Geometry: see drawing. Coordinates: mm, zero at the bounding-box minimum. A direction names the side the tool comes from. Give positions to 0.01 mm unless a question says otherwise; leave off trailing zeros. Order: outer loops, then holes, each group sorted by start corner. A loop starts at its lowest first (then second) coordinate and runs counter-clockwise, first axis right, second up. Notation, with made-up numbers: (-2, 8) - (28, 8) arc R20 cw to (28, 29) - close; hole circle Ø5 at (85.5, 56). An arc over 180 degrees is marked (long way). Put each result on its own line as item: value. Start each with the question number.
1. Set-up query: the marked faces 4, 5 and 6. Return all of +Z, -Z, +X, -X, +Y, -Y with unobstructed straight access to the full face (end or side cutting, diameter ignored); none if empty.
2. Section D-D on y = 4.6. Return the cut outline in (x, z) (1 decimal).
3. Mould query, pull axis Y, two halves, no side actions, for the marked faces 1, 2 and 3. Classes: pulls with the +Y half, pulls with the -Y half, needs draft (parallel to the pull), parting line crosses it, or undercut.
4. Section C-C on z = 7.25. Return the cut outline in (x, y).
5. Ray query, line 1 along Z through (x, y) = (4.5, 1.9); line 2 along Y through (x, z) = (3.55, 11.5); line 3 along Y through (x, z) = (2.4, 12). Return the intervals inside material, ascending. Write a range as from..to.
6. Section B-B on x = 3.1. Return the cut outline in (y, z).
7. First-contact query: P1, Ø2, axis at y = 4, z = 8, coming from the -X side; P2, Ø1.5, axis at y = 1, z = 11.5, coming from the +X side. Flat tips, straight axial feed; report the tip coordinate or a pass-through.
8. Section A-A on y = 2.75. Return the cut outline in (x, z).
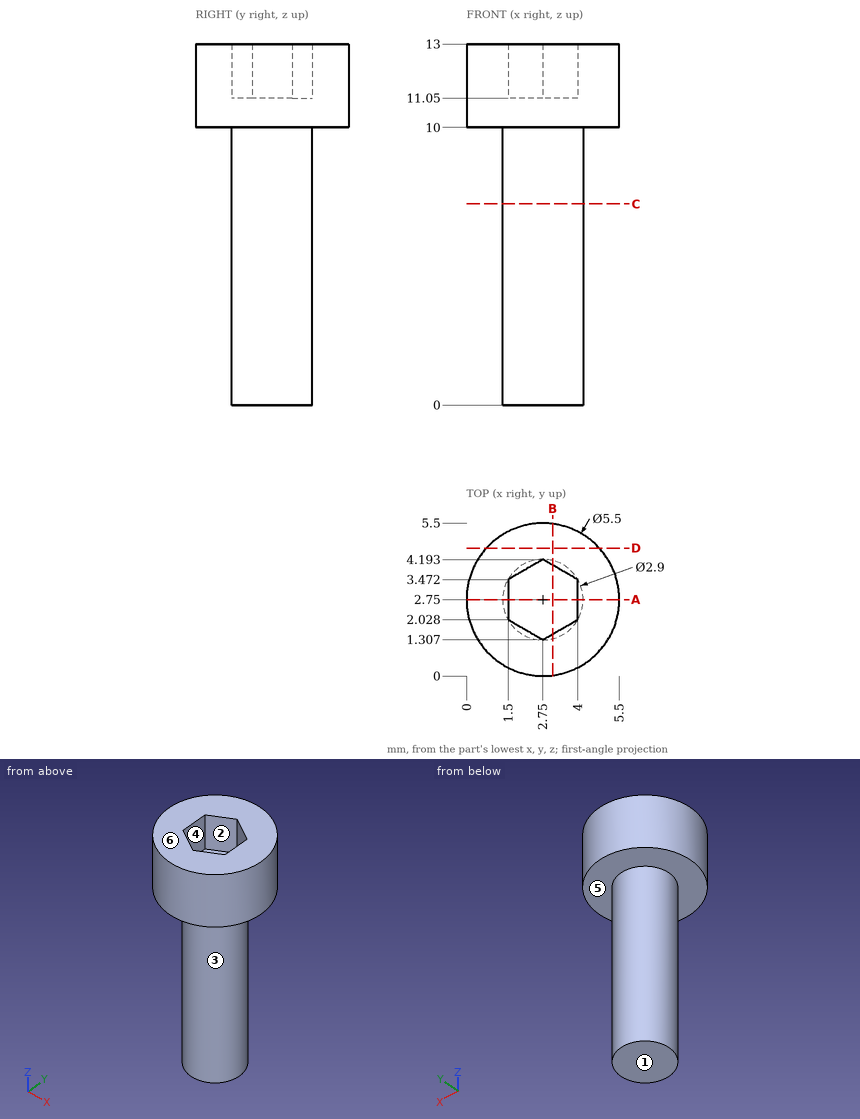
Resolved:
1. face 4: +Z
1. face 5: -Z
1. face 6: +Z, +X, -X, +Y, -Y
2. outline: (0.7, 10) - (4.8, 10) - (4.8, 13) - (0.7, 13) - close
3. face 1: needs draft
3. face 2: undercut
3. face 3: parting line crosses it
4. outline: circle Ø2.9 at (2.75, 2.75)
5. line 1: 10..13
5. line 2: 0.12..1.77, 3.73..5.38
5. line 3: 0.02..1.51, 3.99..5.48
6. outline: (0.02, 10) - (1.34, 10) - (1.34, 0) - (4.16, 0) - (4.16, 10) - (5.48, 10) - (5.48, 13) - (3.99, 13) - (3.99, 11.05) - (1.51, 11.05) - (1.51, 13) - (0.02, 13) - close
7. P1: x = 1.32
7. P2: x = 5.31
8. outline: (0, 10) - (1.3, 10) - (1.3, 0) - (4.2, 0) - (4.2, 10) - (5.5, 10) - (5.5, 13) - (4, 13) - (4, 11.05) - (1.5, 11.05) - (1.5, 13) - (0, 13) - close
